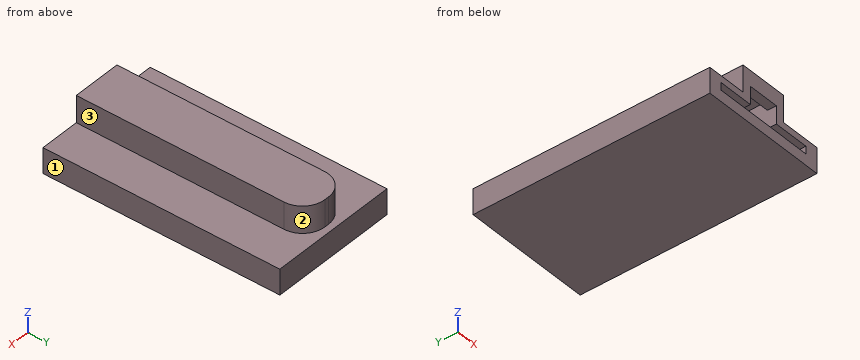
```python
from build123d import *

# Parameters (mm, degrees)
F0_W      = 23
F0_H      = 50
F1_DEPTH  = 1.5
F2_DEPTH  = 3.2
F3_W      = 7
F3_H      = 3
F3_W_2    = 6
F3_H_2    = 50
F4_DEPTH  = 1.5
F3_W_3    = 2
F5_DEPTH  = 6
F6_W      = 11
F6_H      = 1.5
F7_DEPTH  = 4.5
F8_W      = 11
F8_H      = 51.5
F9_DEPTH  = 1.5
F10_R     = 5
F11_W     = 29
F11_H     = 53
F12_DEPTH = 1
F13_W     = 7
F13_H     = 2
F14_DEPTH = 2


with BuildPart() as f1:
    # F0 (on Top) → F1 (new body)
    with BuildSketch(Plane.XY):
        with Locations((-14.5, -16.2683480976)):
            Rectangle(F0_W, F0_H)
    extrude(amount=F1_DEPTH)

    # F0 (on Top) → F2 (join)
    with BuildSketch(Plane.XY):
        Polygon((-26, -41.2683480976), (-26, 8.7316519024), (-3, 8.7316519024), (-3, -41.2683480976), (0, -41.2683480976), (0, 11.7316519024), (-29, 11.7316519024), (-29, -41.2683480976), align=None)
    extrude(amount=F2_DEPTH)

    # F3 (on face) → F4 (join)
    with BuildSketch(Plane.XY.offset(3.2)):
        with Locations((-14.5, 10.2316519024)):
            Rectangle(F3_W, F3_H)
        with Locations((-23, -16.2683480976)):
            Rectangle(F3_W_2, F3_H_2)
        with Locations((-6, -16.2683480976)):
            Rectangle(F3_W_2, F3_H_2)
        Polygon((-18, 11.7316519024), (-29, 11.7316519024), (-29, -41.2683480976), (-26, -41.2683480976), (-26, 8.7316519024), (-20, 8.7316519024), (-18, 8.7316519024), align=None)
        Polygon((0, 11.7316519024), (-11, 11.7316519024), (-11, 8.7316519024), (-9, 8.7316519024), (-3, 8.7316519024), (-3, -41.2683480976), (0, -41.2683480976), align=None)
    extrude(amount=F4_DEPTH)

    # F3 (on face) → F5 (join)
    with BuildSketch(Plane.XY.offset(3.2)):
        with Locations((-10, -16.2683480976)):
            Rectangle(F3_W_3, F3_H_2)
        with Locations((-19, -16.2683480976)):
            Rectangle(F3_W_3, F3_H_2)
    extrude(amount=F5_DEPTH)

    # F6 (on face) → F7 (join)
    with BuildSketch(Plane.XY.offset(4.7)):
        with Locations((-14.5, 9.4816519024)):
            Rectangle(F6_W, F6_H)
    extrude(amount=F7_DEPTH)

    # F8 (on face) → F9 (join)
    with BuildSketch(Plane.XY.offset(9.2)):
        with Locations((-14.5, -15.5183480976)):
            Rectangle(F8_W, F8_H)
    extrude(amount=F9_DEPTH)

    # F10
    f10_edges = [f1.edges().sort_by_distance(p)[0] for p in [
        (-20, 10.231652, 7.7),
        (-9, 10.231652, 7.7),
    ]]
    fillet(f10_edges, radius=F10_R)

    # F11 (on face) → F12 (join)
    with BuildSketch(Plane(origin=(0, 0, 0), x_dir=(1, 0, 0), z_dir=(0, 0, -1))):
        with Locations((-14.5, 14.7683480976)):
            Rectangle(F11_W, F11_H)
    extrude(amount=F12_DEPTH)

    # F13 (on face) → F14 (join)
    with BuildSketch(Plane(origin=(0, 0, 9.2), x_dir=(1, 0, 0), z_dir=(0, 0, -1))):
        with Locations((-14.5, 40.2683480976)):
            Rectangle(F13_W, F13_H)
    extrude(amount=F14_DEPTH)


solid = f1.part
```
The model under review builds one solid part; all positions refer to its coordinate system, in mm. Face numbers are marked on the shaded views. A direction names the side the tool comes from. Round coordinates to 2 decimals unless told otherwise and drop trailing zeros. Write each loop counter-clockwise with the first axis right and the second up, starting at its lowest first coordinate (ties: lowest second). Pieces come first, ordered by that corner, then holes. Notation, with made-up numbers: (45, 16) -> (95, 16) arc R27 cw to (95, 46) -> close; hole circle Ø6 at (73, 13). An arc over 180 degrees is marked (long way). Use CSV: the item, a comma, the result in double quotes.
Q1. Consider section D-D (x = -15.75). Give the boundary of the cut face in (y, z), then the cut area to 3 significant figures.
Checks:
outline,"(-41.27, -1) -> (11.73, -1) -> (11.73, 4.7) -> (10.18, 4.7) -> (10.18, 10.7) -> (-41.27, 10.7) -> (-41.27, 7.2) -> (-39.27, 7.2) -> (-39.27, 9.2) -> (8.73, 9.2) -> (8.73, 1.5) -> (-41.27, 1.5) -> close"
area,"230 mm²"
Q2. Consider section B-B (y = -17.5). Give the boundary of the cut face in (x, z), then the cut area to 3 significant figures.
Checks:
outline,"(-29, -1) -> (0, -1) -> (0, 4.7) -> (-9, 4.7) -> (-9, 10.7) -> (-20, 10.7) -> (-20, 4.7) -> (-29, 4.7) -> close; hole (-26, 1.5) -> (-3, 1.5) -> (-3, 3.2) -> (-11, 3.2) -> (-11, 9.2) -> (-18, 9.2) -> (-18, 3.2) -> (-26, 3.2) -> close"
area,"150 mm²"
Q3. For the marked faces 1, 2 and 3, list the 3-axis set-ups (+Z, -Z, +X, -X, +Y, -Y) from which the entire face can be reached by the end or side of a thin tool; tool diameter is ignored.
Checks:
face 1,"+Z, -Z, +X, +Y, -Y"
face 2,"+Z, +X, +Y"
face 3,"+Z, +X, +Y, -Y"
Q4. To check wall thickness, follow probe 1 along X at (y, z) = (-15, 7.75); probe 2 along Z at (x, y) = (-19.5, -16); probe 3 along Z at (x, y) = (-3.75, -13). State the ranges of each line that lie inside material, in increasing order. Write a range as [from, to].
Checks:
probe 1,"[-20, -18], [-11, -9]"
probe 2,"[-1, 1.5], [3.2, 10.7]"
probe 3,"[-1, 1.5], [3.2, 4.7]"
Q5. For pin 1 Ø6 at (x, z) = (-14, 4) entering from -Y; pin 2 Ø6.5 at (y, z) = (-26.5, 8) entering from +X; pin 3 Ø2 at (y, z) = (-18, 8.5) entering from -X; pin 4 Ø2 at (x, z) = (-14, 8.5) entering from +Y, all flat-tipped, find the tip position at first contact; note any pin that passes through.
Checks:
pin 1,"y = -41.27"
pin 2,"x = -9"
pin 3,"x = -20"
pin 4,"y = 10.23"
Q6. Consider section C-C (z = 8.5). Give the boundary of the cut face in (x, y), then the cut area to 3 significant figures.
Checks:
outline,"(-20, -41.27) -> (-9, -41.27) -> (-9, 5.23) arc R5 ccw to (-14, 10.23) -> (-15, 10.23) arc R5 ccw to (-20, 5.23) -> close; hole (-18, -39.27) -> (-11, -39.27) -> (-11, 8.73) -> (-18, 8.73) -> close"
area,"220 mm²"
Q7. Consider section A-A (z = 2.25). Give the boundary of the cut face in (x, y), then the cut area to 3 significant figures.
Checks:
outline,"(-29, -41.27) -> (-26, -41.27) -> (-26, 8.73) -> (-3, 8.73) -> (-3, -41.27) -> (0, -41.27) -> (0, 11.73) -> (-29, 11.73) -> close"
area,"387 mm²"
